CAD build for the part. Positions are in the model's coordinates, mm. A direction names the side the tool comes from. Give positions to 0.01 mm unless a question says otherwise; leave off trailing zeros. Loops run counter-clockwise (first coordinate to the right, second up) from the corner with the lowest first, then second, coordinate; pieces in that order, holes last. Notation, with made-up numbers: M 21.5,87 L 62.5,87 A12 ccw 62.5,96 Z; hole C 32,-28 d8. An arc over 180 degrees is marked long. Answer as CSV lines item,"result".
```python
from build123d import *

# Parameters (mm, degrees)
SKETCH1_W          = 156
SKETCH1_H          = 196
BASE_FLANGE1_DEPTH = 0.5
EDGE_FLANGE1_DEPTH = 196
EDGE_FLANGE2_DEPTH = 156
EDGE_FLANGE3_DEPTH = 196
EDGE_FLANGE4_DEPTH = 156
SKETCH14_W         = 22
SKETCH14_H         = 180
CUT_EXTRUDE1_DEPTH = 2
SKETCH15_R         = 2
CUT_EXTRUDE2_DEPTH = 2


# Sheet-metal steps are written as plain solids
with BuildPart() as part:
    # Sketch1 → Base-Flange1 (new body)
    with BuildSketch(Plane(origin=(0, 0, 0), x_dir=(1, 0, 0), z_dir=(0, 1, 0))):
        with Locations((78, -98)):
            Rectangle(SKETCH1_W, SKETCH1_H)
    extrude(amount=-BASE_FLANGE1_DEPTH)

    # Edge-Flange1 section (across the edge) → Edge-Flange1 (add)
    with BuildSketch(Plane(origin=(-1, 0, 0), x_dir=(1, 0, 0), z_dir=(0, 0, 1))):
        with BuildLine():
            Line((-0.5, 1), (-0.5, 12))
            Line((-0.5, 12), (0, 12))
            Line((0, 12), (0, 1))
            ThreePointArc((0, 1), (0.292893219, 0.292893219), (1, 0))
            Line((1, 0), (1, -0.5))
            ThreePointArc((1, -0.5), (-0.060660172, -0.060660172), (-0.5, 1))
        make_face()
    extrude(amount=EDGE_FLANGE1_DEPTH)

    # Edge-Flange2 section (across the edge) → Edge-Flange2 (add)
    with BuildSketch(Plane(origin=(0, 0, 197), x_dir=(0, 0, -1), z_dir=(1, 0, 0))):
        with BuildLine():
            Line((-0.5, 1), (-0.5, 12))
            Line((-0.5, 12), (0, 12))
            Line((0, 12), (0, 1))
            ThreePointArc((0, 1), (0.292893219, 0.292893219), (1, 0))
            Line((1, 0), (1, -0.5))
            ThreePointArc((1, -0.5), (-0.060660172, -0.060660172), (-0.5, 1))
        make_face()
    extrude(amount=EDGE_FLANGE2_DEPTH)

    # Edge-Flange3 section (across the edge) → Edge-Flange3 (add)
    with BuildSketch(Plane(origin=(157, 0, 196), x_dir=(-1, 0, 0), z_dir=(0, 0, -1))):
        with BuildLine():
            Line((-0.5, 1), (-0.5, 12))
            Line((-0.5, 12), (0, 12))
            Line((0, 12), (0, 1))
            ThreePointArc((0, 1), (0.292893219, 0.292893219), (1, 0))
            Line((1, 0), (1, -0.5))
            ThreePointArc((1, -0.5), (-0.060660172, -0.060660172), (-0.5, 1))
        make_face()
    extrude(amount=EDGE_FLANGE3_DEPTH)

    # Edge-Flange4 section (across the edge) → Edge-Flange4 (add)
    with BuildSketch(Plane(origin=(156, 0, -1), x_dir=(0, 0, 1), z_dir=(-1, 0, 0))):
        with BuildLine():
            Line((-0.5, 1), (-0.5, 12))
            Line((-0.5, 12), (0, 12))
            Line((0, 12), (0, 1))
            ThreePointArc((0, 1), (0.292893219, 0.292893219), (1, 0))
            Line((1, 0), (1, -0.5))
            ThreePointArc((1, -0.5), (-0.060660172, -0.060660172), (-0.5, 1))
        make_face()
    extrude(amount=EDGE_FLANGE4_DEPTH)

    # Sketch14 → Cut-Extrude1 (cut)
    with BuildSketch(Plane.XZ.offset(0.5)):
        with Locations((78, 98.144635834)):
            Rectangle(SKETCH14_W, SKETCH14_H)
    extrude(amount=-CUT_EXTRUDE1_DEPTH, mode=Mode.SUBTRACT)

    # Sketch15 → Cut-Extrude2 (cut)
    with BuildSketch(Plane(origin=(0, 0, 0), x_dir=(1, 0, 0), z_dir=(0, 1, 0))):
        with Locations(Location((93.6217, -175.805181717, 0), (0, 0, 270))):
            Circle(SKETCH15_R)
        with Locations(Location((62.3851, -175.805181717, 0), (0, 0, 270))):
            Circle(SKETCH15_R)
        with Locations(Location((93.6217, -126.552336837, 0), (0, 0, 270))):
            Circle(SKETCH15_R)
        with Locations(Location((62.3851, -126.552336837, 0), (0, 0, 270))):
            Circle(SKETCH15_R)
        with Locations(Location((93.6217, -68.939033602, 0), (0, 0, 270))):
            Circle(SKETCH15_R)
        with Locations(Location((62.3851, -68.939033602, 0), (0, 0, 270))):
            Circle(SKETCH15_R)
        with Locations(Location((93.6217, -19.686188722, 0), (0, 0, 270))):
            Circle(SKETCH15_R)
        with Locations(Location((62.3851, -19.686188722, 0), (0, 0, 270))):
            Circle(SKETCH15_R)
    extrude(amount=-CUT_EXTRUDE2_DEPTH, mode=Mode.SUBTRACT)


solid = part.part
```
Q1. Wall check: line 1 (Z direction, x = 6, y = 0.75); line 2 (X direction, y = 9, z = 111.5); line 3 (Y direction, x = 20, z = 26.5). Give the ranges that are in metal, low to high. Write a range as [from, to].
Solution:
line 1,"z = [-1.48, -0.97], [196.97, 197.48]"
line 2,"x = [-1.5, -1], [157, 157.5]"
line 3,"y = [-0.5, 0]"
Q2. Pin check, flat tips, straight feed: P1, Ø1.2, axis at y = 8.5, z = 197, coming from the +X side; P2, Ø5, axis at x = 93.62, z = 68.94, coming from the +Y side; P3, Ø1.6, axis at x = 156.5, y = 4.5, coming from the +Z side; P4, Ø0.8, axis at x = 157, y = 3, coming from the -Z side. Stop position of each tip, or through.
Solution:
P1,"stops at x = 156"
P2,"stops at y = 0"
P3,"stops at z = 197.5"
P4,"stops at z = 0"
Q3. Cut at A-A (y = 7.75). Write the cut outline in (x, z).
Solution:
outline,"M -1.5,0 L -1,0 L -1,196 L -1.5,196 Z; M 0,-1.5 L 156,-1.5 L 156,-1 L 0,-1 Z; M 0,197 L 156,197 L 156,197.5 L 0,197.5 Z; M 157,0 L 157.5,0 L 157.5,196 L 157,196 Z"
Q4. Mould opens along X. For faces 5 (the cylindrical face through (60.61, -0.25, 20.61)), 6 (the flat face through (157.5, 6, 99)), 7 (the cylindrical face through (61.17, -0.25, 67.35)), 8 (the flat face through (-1.5, 6, 97)) say: released by +X, released by -X, zero draft, split by the parting line, or undercut.
Solution:
face 5,"undercut"
face 6,"released by +X"
face 7,"undercut"
face 8,"released by -X"
Q5. Which spindle directions (+Z, -Z, +X, -X, +Y, -Y) get a long thin tool onto all of the face, cutting with end or side? Do faces 1 (the flat face through (79, 7, -1)), 2 (the flat face through (79, 6, -1.5)), 3 (the flat face through (94, 0, 97)), 4 (the flat face through (-1, 7, 97)). Say none if no direction does.
Solution:
face 1,"+X, -X, +Y"
face 2,"-Z, +X, -X, +Y, -Y"
face 3,"+Y"
face 4,"+Z, -Z, +Y"
Q6. Cut at B-B (z = 38). Write the cut outline in (x, y).
Solution:
outline,"M -1.5,1 A1.5 ccw 0,-0.5 L 67,-0.5 L 67,0 L 0,0 A1 cw -1,1 L -1,12 L -1.5,12 Z; M 89,-0.5 L 156,-0.5 A1.5 ccw 157.5,1 L 157.5,12 L 157,12 L 157,1 A1 cw 156,0 L 89,0 Z"
Q7. Cut at C-C (x = 21). Write the cut outline in (y, z), and give its area (3 significant figures).
Solution:
outline,"M -0.5,0 A1.5 ccw 1,-1.5 L 12,-1.5 L 12,-1 L 1,-1 A1 cw 0,0 L 0,196 A1 cw 1,197 L 12,197 L 12,197.5 L 1,197.5 A1.5 ccw -0.5,196 Z"
area,"111 mm²"
